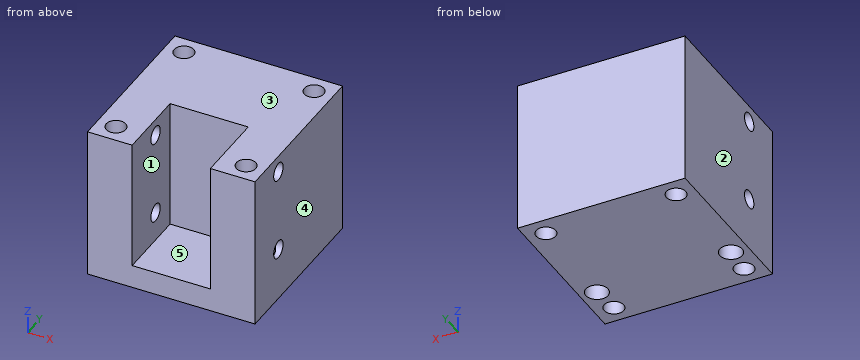
```python
from build123d import *

# Parameters (mm, degrees)
F0_W      = 30
F0_H      = 30
F1_DEPTH  = 27.5
F2_R      = 1.75
F3_DEPTH  = 27.501
F4_R      = 2
F5_DEPTH  = 20
F6_R      = 2
F7_W      = 14
F7_H      = 13
F8_DEPTH  = 23.3
F9_R      = 1.6
F10_DEPTH = 30.001


# Not quite as in the source:
# - a feature names something its author has since deleted; it is built from what else it names


with BuildPart() as f1:
    # F0 (on Top) → F1 (new body)
    with BuildSketch(Plane.XY):
        Rectangle(F0_W, F0_H)
    extrude(amount=F1_DEPTH)

    # F2 (on face) → F3 (cut, through all)
    with BuildSketch(Plane.XY.offset(27.5)):
        with Locations((-11.65, 11.65)):
            Circle(F2_R)
        with Locations((-11.65, -11.65)):
            Circle(F2_R)
        with Locations((11.65, 11.65)):
            Circle(F2_R)
        with Locations((11.65, -11.65)):
            Circle(F2_R)
    extrude(amount=-F3_DEPTH, mode=Mode.SUBTRACT)

    # F4 (on face) → F5 (cut)
    with BuildSketch(Plane(origin=(0, 0, 0), x_dir=(1, 0, 0), z_dir=(0, 0, -1))):
        with Locations((-11.95, 6.6)):
            Circle(F4_R)
        with Locations((12.05, 6.6)):
            Circle(F4_R)
    extrude(amount=-F5_DEPTH, mode=Mode.SUBTRACT)

    # F6
    f6_edges = [f1.edges().sort_by_distance(p)[0] for p in [
        (-13.95, -6.6, 20),
        (10.05, -6.6, 20),
    ]]
    fillet(f6_edges, radius=F6_R)

    # F7 (on face) → F8 (cut)
    with BuildSketch(Plane.XY.offset(27.5)):
        with Locations((0, -8.5)):
            Rectangle(F7_W, F7_H)
    extrude(amount=-F8_DEPTH, mode=Mode.SUBTRACT)

    # F9 (on face) → F10 (cut, through all)
    with BuildSketch(Plane(origin=(-15, 0, 0), x_dir=(0, -1, 0), z_dir=(-1, 0, 0))):
        with Locations((7, 9.5)):
            Circle(F9_R)
        with Locations((7, 24.5)):
            Circle(F9_R)
    extrude(amount=-F10_DEPTH, mode=Mode.SUBTRACT)


solid = f1.part
```
CAD build for the part. Positions are in the model's coordinates, mm. Face numbers are marked on the shaded views. A direction names the side the tool comes from. Round coordinates to 2 decimals unless told otherwise and drop trailing zeros. Order: outer loops, then holes, each group sorted by start corner. A loop starts at its lowest first (then second) coordinate and runs counter-clockwise, first axis right, second up. Notation, with made-up numbers: (1, -12.75) - (38, -12.75) arc R26 ccw to (38, 1.25) - close; hole circle Ø6 at (-10, 66). An arc over 180 degrees is marked (long way). Answer as CSV lines item,"result". Start each with the question number.
1. Pull direction X, two halves, no side cores. Call the marked faces 3, 4 and 5: +X half, -X half, draft (parallel to the pull), parting line (faces both ways), or undercut.
2. Tool access for the marked faces 1 and 2: list every direction of +Z, -Z, +X, -X, +Y, -Y with a clear straight run to the whole face (end or side of a thin tool).
3. Saw through at C-C, the plane z = 14.75. Write the cut outline in (x, y).
4. Saw through at A-A, the plane y = -11.65. Write the cut outline in (x, z), and give its area (3 significant figures).
5. Pin check, flat tip, straight feed: pin 1 (7 mm diameter, centred on x = 1.5, z = 13, fed in from -Y). Stop position of the tip, or through.
6. Saw through at B-B, the plane z = 10. Write the cut outline in (x, y), and give its area (3 significant figures).
7. Drill centre lines: L1, parallel to X at y = -6.6, z = 4; L2, parallel to X at y = -6.6, z = 6; L3, parallel to Y at x = -11.65, z = 22. Where is each one in solid material? Low to high. Write a range as [from, to].
8. Saw through at D-D, the plane x = 4.5. Write the cut outline in (y, z), and give its area (3 significant figures).
Model answer:
1,face 3,"draft"
1,face 4,"+X half"
1,face 5,"undercut"
2,face 1,"+Z, -Y"
2,face 2,"+Z, -Z, -X, +Y, -Y"
3,outline,"(-15, -15) - (-7, -15) - (-7, -2) - (7, -2) - (7, -15) - (15, -15) - (15, 15) - (-15, 15) - close; hole circle Ø4 at (-11.95, -6.6); hole circle Ø3.5 at (-11.65, -11.65); hole circle Ø3.5 at (-11.65, 11.65); hole circle Ø3.5 at (11.65, -11.65); hole circle Ø3.5 at (11.65, 11.65); hole circle Ø4 at (12.05, -6.6)"
4,outline,"(-15, 0) - (-13.4, 0) - (-13.4, 27.5) - (-15, 27.5) - close; (-9.9, 0) - (9.9, 0) - (9.9, 27.5) - (7, 27.5) - (7, 4.2) - (-7, 4.2) - (-7, 27.5) - (-9.9, 27.5) - close; (13.4, 0) - (15, 0) - (15, 27.5) - (13.4, 27.5) - close"
4,area,"306 mm²"
5,pin 1,"stops at y = -2"
6,outline,"(-15, -15) - (-7, -15) - (-7, -8.52) - (-11.39, -8.52) arc R2 cw to (-12.51, -8.52) - (-15, -8.52) - close; (-15, -5.48) - (-13.61, -5.48) arc R2 cw to (-10.29, -5.48) - (-7, -5.48) - (-7, -2) - (7, -2) - (7, -5.48) - (10.39, -5.48) arc R2 cw to (13.71, -5.48) - (15, -5.48) - (15, 15) - (-15, 15) - close; (7, -15) - (15, -15) - (15, -8.52) - (12.61, -8.52) arc R2 cw to (11.49, -8.52) - (7, -8.52) - close; hole circle Ø3.5 at (-11.65, -11.65); hole circle Ø3.5 at (-11.65, 11.65); hole circle Ø3.5 at (11.65, -11.65); hole circle Ø3.5 at (11.65, 11.65)"
6,area,"627 mm²"
7,L1,"x = [-15, -13.95], [-9.95, 10.05], [14.05, 15]"
7,L2,"x = [-15, -13.95], [-9.95, -7], [7, 10.05], [14.05, 15]"
7,L3,"y = [-15, -13.4], [-9.9, 9.9], [13.4, 15]"
8,outline,"(-15, 0) - (15, 0) - (15, 27.5) - (-2, 27.5) - (-2, 4.2) - (-15, 4.2) - close"
8,area,"522 mm²"
